from build123d import *

# Parameters (mm, degrees)
BOSS_EXTRUDE1_DEPTH = 12.7
SKETCH3_R           = 3.81
BOSS_EXTRUDE2_DEPTH = 2.54
BOSS_EXTRUDE2_TAPER = 5
BOSS_EXTRUDE3_START = -38.1
BOSS_EXTRUDE3_DEPTH = 12.7
SKETCH6_R           = 3.81
BOSS_EXTRUDE4_DEPTH = 2.54
BOSS_EXTRUDE4_TAPER = 5
SKETCH7_W           = 12.7
SKETCH7_H           = 6.172188314
BOSS_EXTRUDE5_DEPTH = 63.5
SKETCH8_W           = 15.24
SKETCH8_H           = 12.7
BOSS_EXTRUDE6_DEPTH = 5.08
SKETCH9_R           = 2.5
CUT_EXTRUDE3_DEPTH  = 5.08
FILLET6_R           = 2.54


with BuildPart() as part:
    # Sketch2 → Boss-Extrude1 (new body)
    with BuildSketch(Plane.XY):
        with BuildLine():
            Line((-31.75, -26.67), (31.75, -26.67))
            Line((31.75, -26.67), (31.75, -20.497811686))
            Line((31.75, -20.497811686), (21.297259116, -13.749518324))
            ThreePointArc((21.297259116, -13.749518324), (24.315715274, -7.167181503), (25.35, 0))
            Line((25.35, 0), (19, 0))
            ThreePointArc((19, 0), (0, -19), (-19, 0))
            Line((-19, 0), (-25.35, 0))
            ThreePointArc((-25.35, 0), (-24.315715274, -7.167181503), (-21.297259116, -13.749518324))
            Line((-21.297259116, -13.749518324), (-31.75, -20.497811686))
            Line((-31.75, -20.497811686), (-31.75, -26.67))
        make_face()
    extrude(amount=BOSS_EXTRUDE1_DEPTH)

    # Sketch3 → Boss-Extrude2 (add)
    with BuildSketch(Plane.XZ.offset(26.67)):
        with Locations((-25.4, 6.35)):
            Circle(SKETCH3_R)
        with Locations((25.4, 6.35)):
            Circle(SKETCH3_R)
    extrude(amount=BOSS_EXTRUDE2_DEPTH, taper=BOSS_EXTRUDE2_TAPER)



with BuildPart() as body_2:
    # Sketch2_2 → Boss-Extrude3 (new body)
    with BuildSketch(Plane.XY.offset(BOSS_EXTRUDE3_START)):
        with BuildLine():
            Line((-31.75, -26.67), (31.75, -26.67))
            Line((31.75, -26.67), (31.75, -20.497811686))
            Line((31.75, -20.497811686), (21.297259116, -13.749518324))
            ThreePointArc((21.297259116, -13.749518324), (24.315715274, -7.167181503), (25.35, 0))
            Line((25.35, 0), (19, 0))
            ThreePointArc((19, 0), (0, -19), (-19, 0))
            Line((-19, 0), (-25.35, 0))
            ThreePointArc((-25.35, 0), (-24.315715274, -7.167181503), (-21.297259116, -13.749518324))
            Line((-21.297259116, -13.749518324), (-31.75, -20.497811686))
            Line((-31.75, -20.497811686), (-31.75, -26.67))
        make_face()
    extrude(amount=-BOSS_EXTRUDE3_DEPTH)

    # Sketch6 → Boss-Extrude4 (add)
    with BuildSketch(Plane.XZ.offset(26.67)):
        with Locations((-25.4, -44.45)):
            Circle(SKETCH6_R)
        with Locations((25.4, -44.45)):
            Circle(SKETCH6_R)
    extrude(amount=BOSS_EXTRUDE4_DEPTH, taper=BOSS_EXTRUDE4_TAPER)


with BuildPart() as part_1:
    add(part.part)

    add(body_2.part)  # Boss-Extrude5 merges body 2
    # Sketch7 → Boss-Extrude5 (add, through all)
    with BuildSketch(Plane.XY.offset(12.7)):
        with Locations((-25.4, -23.583905843)):
            Rectangle(SKETCH7_W, SKETCH7_H)
        with Locations((25.4, -23.583905843)):
            Rectangle(SKETCH7_W, SKETCH7_H)
    extrude(amount=-BOSS_EXTRUDE5_DEPTH)

    # Sketch8 → Boss-Extrude6 (add)
    with BuildSketch(Plane(origin=(0, 0, 0), x_dir=(1, 0, 0), z_dir=(0, 1, 0))):
        with Locations((26.62, -6.35)):
            Rectangle(SKETCH8_W, SKETCH8_H)
        with Locations((-26.62, 44.45)):
            Rectangle(SKETCH8_W, SKETCH8_H)
        with Locations((26.62, 44.45)):
            Rectangle(SKETCH8_W, SKETCH8_H)
        with Locations((-26.62, -6.35)):
            Rectangle(SKETCH8_W, SKETCH8_H)
    extrude(amount=-BOSS_EXTRUDE6_DEPTH)

    # Sketch9 → Cut-Extrude3 (cut)
    with BuildSketch(Plane(origin=(0, -5.08, 0), x_dir=(-1, 0, 0), z_dir=(0, -1, 0))):
        with Locations((30.43, 44.45)):
            Circle(SKETCH9_R)
        with Locations((-30.43, 44.45)):
            Circle(SKETCH9_R)
        with Locations((-30.43, -6.35)):
            Circle(SKETCH9_R)
        with Locations((30.43, -6.35)):
            Circle(SKETCH9_R)
    extrude(amount=-CUT_EXTRUDE3_DEPTH, mode=Mode.SUBTRACT)

    # Fillet6
    fillet6_edges = [part_1.edges().sort_by_distance(p)[0] for p in [
        (-19.05, -20.497811686, -19.05),
        (-31.75, -20.497811686, -19.05),
        (31.75, -20.497811686, -19.05),
        (19.05, -20.497811686, -19.05),
    ]]
    fillet(fillet6_edges, radius=FILLET6_R)


solid = part_1.part
Could you check a few things on this model? Use its own coordinates, in mm. A direction names the side the tool comes from. Give positions to 0.01 mm unless a question says otherwise; leave off trailing zeros. Loops run counter-clockwise (first coordinate to the right, second up) from the corner with the lowest first, then second, coordinate; pieces in that order, holes last. Notation, with made-up numbers: (53, 44) -> (57, 44) arc R15 cw to (57, 71) -> close; hole circle Ø4 at (-35.5, 23.25). An arc over 180 degrees is marked (long way). Return JSON: item names as keys, results as strings.
Item 1: We'd pull the mould along Z, two halves only. Please class faces 1 (the flat face through (34.24, -3, 6)), 2 (the cylindrical face through (-28.59, -2.58, -46.14)): +Z half, -Z half, draft (parallel to the pull), parting line (faces both ways), or undercut.
Geometry results:
{"face 1": "draft", "face 2": "undercut"}
Item 2: If we section it at A-A on y = -8.75: List the corners of the cut face in (x, z) for me, plus the area to 3 significant figures.
Geometry results:
{"outline": "(-23.79, -50.8) -> (-16.87, -50.8) -> (-16.87, -38.1) -> (-23.79, -38.1) -> close; (-23.79, 0) -> (-16.87, 0) -> (-16.87, 12.7) -> (-23.79, 12.7) -> close; (16.87, -50.8) -> (23.79, -50.8) -> (23.79, -38.1) -> (16.87, -38.1) -> close; (16.87, 0) -> (23.79, 0) -> (23.79, 12.7) -> (16.87, 12.7) -> close", "area": "352 mm²"}
Item 3: If we section it at C-C on z = -23.5: List the corners of the cut face in (x, y) for me, plus the area to 3 significant figures.
Geometry results:
{"outline": "(-31.75, -26.67) -> (-19.05, -26.67) -> (-19.05, -23.04) arc R2.54 ccw to (-21.59, -20.5) -> (-29.21, -20.5) arc R2.54 ccw to (-31.75, -23.04) -> close; (19.05, -26.67) -> (31.75, -26.67) -> (31.75, -23.04) arc R2.54 ccw to (29.21, -20.5) -> (21.59, -20.5) arc R2.54 ccw to (19.05, -23.04) -> close", "area": "151 mm²"}
Item 4: I need wall thicknesses on L1, parallel to Z at x = 30.43, y = -1.4; L2, parallel to X at y = -23.5, z = -26; L3, parallel to X at y = -2.15, z = -44.45. Which ranges of each line are inside material? Lowest first, please. Write a range as from..to.
Geometry results:
{"L1": "z = -50.8..-46.95, -41.95..-38.1, 0..3.85, 8.85..12.7", "L2": "x = -31.75..-19.05, 19.05..31.75", "L3": "x = -34.24..-32.93, -27.93..-18.88, 18.88..27.93, 32.93..34.24"}
Item 5: If we section it at D-D on x = -30.43: List the corners of the cut face in (y, z) for me.
Geometry results:
{"outline": "(-26.67, -50.8) -> (-19.65, -50.8) -> (-19.65, -38.1) -> (-20.81, -38.1) -> (-20.81, 0) -> (-19.65, 0) -> (-19.65, 12.7) -> (-26.67, 12.7) -> close; (-5.08, -50.8) -> (0, -50.8) -> (0, -46.95) -> (-5.08, -46.95) -> close; (-5.08, -41.95) -> (0, -41.95) -> (0, -38.1) -> (-5.08, -38.1) -> close; (-5.08, 0) -> (0, 0) -> (0, 3.85) -> (-5.08, 3.85) -> close; (-5.08, 8.85) -> (0, 8.85) -> (0, 12.7) -> (-5.08, 12.7) -> close"}
Item 6: I'm going to push flat-ended pins straight in: pin 1 (3 mm diameter, centred on y = -22.5, z = -32, fed in from -X); pin 2 (8.5 mm diameter, centred on x = -25.5, z = -17.5, fed in from +Y); pin 3 (3 mm diameter, centred on x = -30.43, z = -44.45, fed in from +Y); pin 4 (1.5 mm diameter, centred on x = 26, y = -10.5, fed in from -Z). Where does each tip first touch, or does it pass through?
Geometry results:
{"pin 1": "stops at x = -31.75", "pin 2": "stops at y = -20.5", "pin 3": "stops at y = -18.68", "pin 4": "passes through"}
Item 7: If we section it at B-B on x = 2.5: List the corners of the cut face in (y, z) for me.
Geometry results:
{"outline": "(-26.67, -50.8) -> (-18.83, -50.8) -> (-18.83, -38.1) -> (-26.67, -38.1) -> close; (-26.67, 0) -> (-18.83, 0) -> (-18.83, 12.7) -> (-26.67, 12.7) -> close"}
Item 8: Which directions (+Z, -Z, +X, -X, +Y, -Y) give clear straight access to the entire face, cutting with the end or side of a thin tool? Please do faces 3 (the flat face through (26.597, -17.171, 6.261)), 4 (the flat face through (-25, -20.498, -19)), 5 (the cylindrical face through (31.026, -21.262, -19.317)), 6 (the cylindrical face through (28.12, -2.58, 7.31)).
Geometry results:
{"face 3": "+Z, -Z, +X", "face 4": "+X, -X, +Y", "face 5": "+X, +Y", "face 6": "+Y"}
